Here's the drawing with two shaded views (mm, measured from the low corner). I have some questions. A direction names the side the tool comes from. Round coordinates to 2 decimals unless told otherwise and drop trailing zeros. Loops run counter-clockwise (first coordinate to the right, second up) from the corner with the lowest first, then second, coordinate; pieces in that order, holes last.
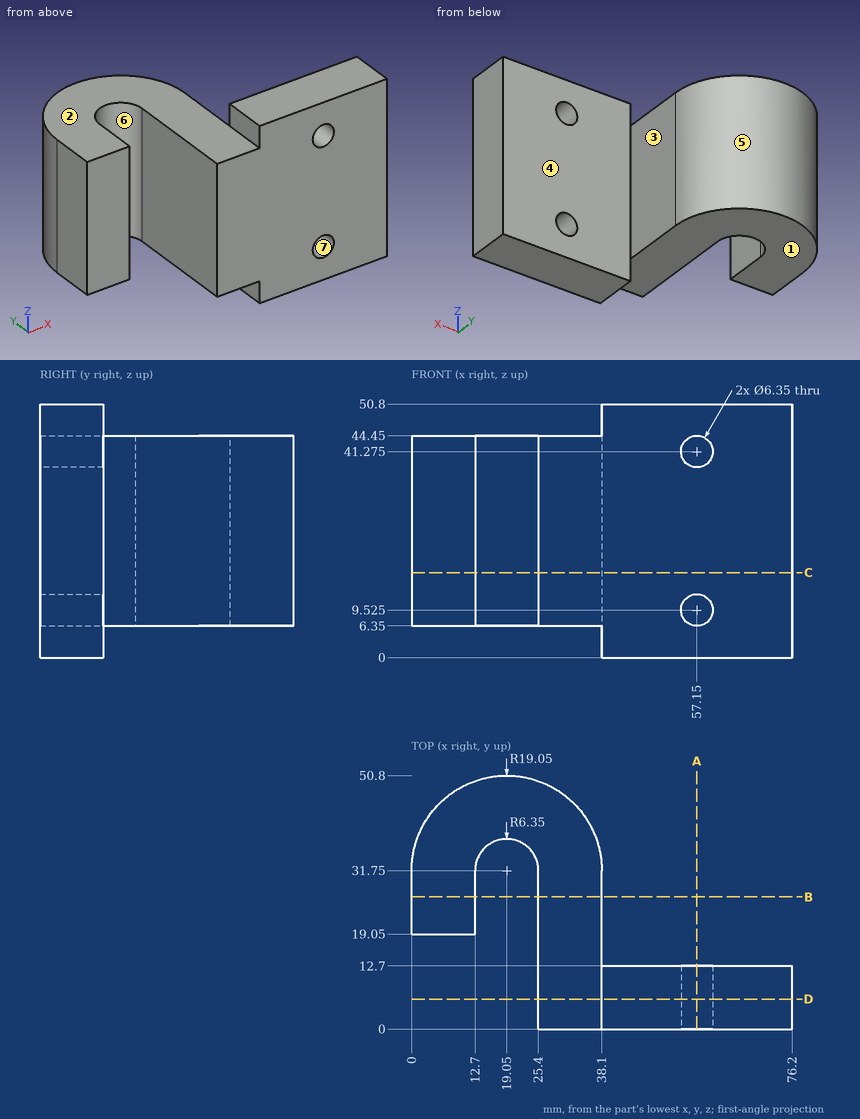
Item 1: For the marked faces 1, 2 and 3, which set-ups out of +Z, -Z, +X, -X, +Y, -Y let a thin tool reach every point of the face, with its end or its side?
Results list:
face 1: -Z, -X, +Y, -Y
face 2: +Z, -X, +Y, -Y
face 3: +Z, -Z, +X, +Y
Item 2: Will these pins go through, and if not, where does the flat tip stop? pin 1 (5.5 mm diameter, centred on y = 24, z = 34.5, fed in from +X); pin 2 (19 mm diameter, centred on x = 20, y = 21.5, fed in from +Z); pin 3 (19 mm diameter, centred on x = 11, y = 24, fed in from -Z).
Results list:
pin 1: stops at x = 38.1
pin 2: stops at z = 44.45
pin 3: stops at z = 6.35
Item 3: If we section it at A-A, the plane x = 57.15: Please give me the cut outline in (y, z), then the cut area to 3 significant figures.
Results list:
outline: (0, 0) - (12.7, 0) - (12.7, 6.35) - (0, 6.35) - close; (0, 12.7) - (12.7, 12.7) - (12.7, 38.1) - (0, 38.1) - close; (0, 44.45) - (12.7, 44.45) - (12.7, 50.8) - (0, 50.8) - close
area: 484 mm2
Item 4: If we section it at B-B, the plane y = 26.5: Please give me the cut outline in (x, z), then the cut area to 3 significant figures.
Results list:
outline: (0, 6.35) - (12.7, 6.35) - (12.7, 44.45) - (0, 44.45) - close; (25.4, 6.35) - (38.1, 6.35) - (38.1, 44.45) - (25.4, 44.45) - close
area: 968 mm2
Item 5: If we section it at D-D, the plane y = 6: Please give me the cut outline in (x, z) (3 decimals), then the cut area to 3 significant figures.
Results list:
outline: (25.4, 6.35) - (38.1, 6.35) - (38.1, 0) - (76.2, 0) - (76.2, 50.8) - (38.1, 50.8) - (38.1, 44.45) - (25.4, 44.45) - close; hole circle Ø6.35 at (57.15, 9.525); hole circle Ø6.35 at (57.15, 41.275)
area: 2,360 mm2
Item 6: If I drill on line 1 along Z through (x, y) = (57, 3); line 2 along X through (y, z) = (23, 15.5); line 3 along X through (y, z) = (14, 18), over which ranges is the centre line in solid material (lowest first)?
Results list:
line 1: z = 0 to 6.35, 12.7 to 38.1, 44.45 to 50.8
line 2: x = 0 to 12.7, 25.4 to 38.1
line 3: x = 25.4 to 38.1
Item 7: If we section it at C-C, the plane z = 17: Please give me the cut outline in (x, y), then the cut area to 3 significant figures.
Results list:
outline: (0, 19.05) - (12.7, 19.05) - (12.7, 31.75) arc R6.35 cw to (25.4, 31.75) - (25.4, 0) - (76.2, 0) - (76.2, 12.7) - (38.1, 12.7) - (38.1, 31.75) arc R19.05 ccw to (0, 31.75) - close
area: 1,560 mm2
Item 8: We'd pull the mould along X, two halves only. Please class the marked faces 4, 5, 6 and 7: released by +X, released by -X, zero draft, split by the parting line, or undercut.
Results list:
face 4: zero draft
face 5: split by the parting line
face 6: undercut
face 7: undercut
